Check sheet for the drawn part. Datum: minimum x, y, z corner. Units: mm. A direction names the side the tool comes from. Round coordinates to 2 decimals unless told otherwise and drop trailing zeros. Order: outer loops, then holes, each group sorted by start corner. A loop starts at its lowest first (then second) coordinate and runs counter-clockwise, first axis right, second up. Notation, with made-up numbers: (58.5, 32) -> (102.5, 32) arc R18 cw to (102.5, 40) -> close; hole circle Ø9 at (59.5, 53.5). An arc over 180 degrees is marked (long way). Answer as CSV lines item,"result". Start each with the question number.
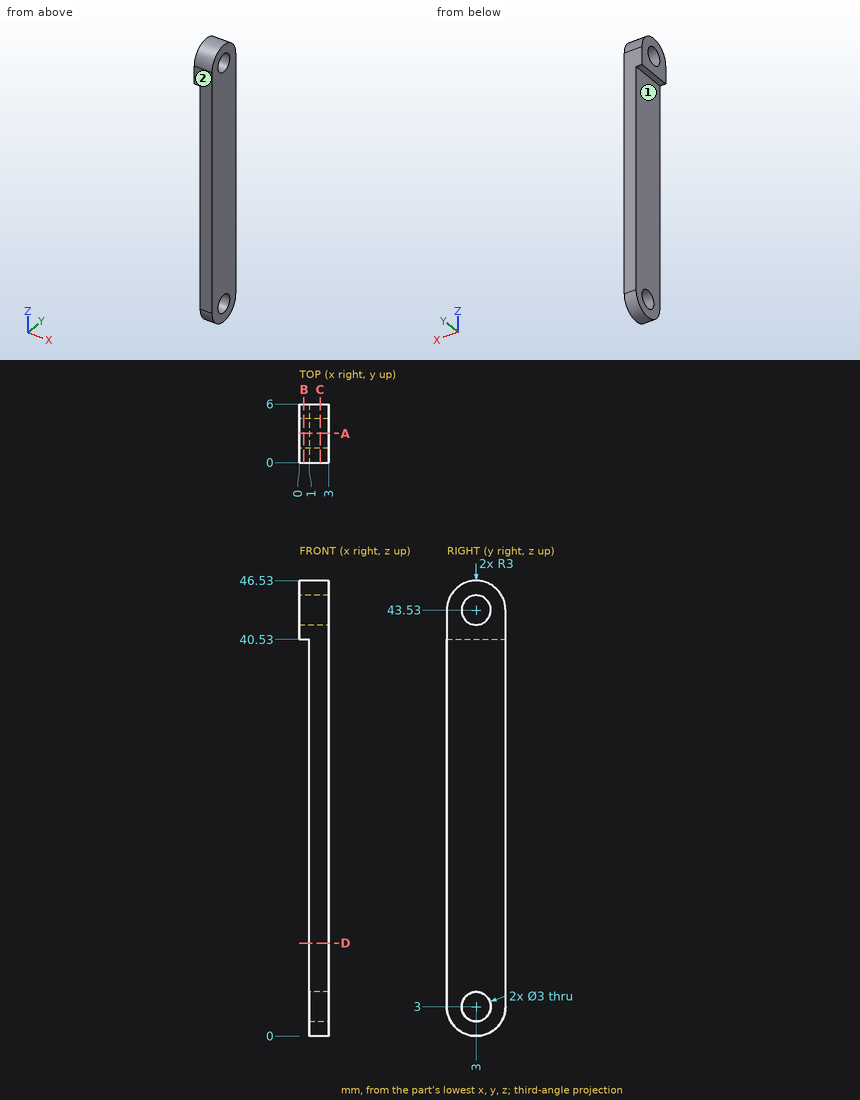
1) Section check A-A on y = 3. Record the cut outline in (x, z), then the cut area to 3 significant figures.
2) Section check B-B on x = 0.45. Record the cut outline in (y, z), then the cut area to 3 significant figures.
3) Depth check by flat-ended pin: pin 1 Ø1 at (x, y) = (1, 1) entering from +Z; pin 2 Ø1.8 at (y, z) = (1.5, 11) entering from -X. Enter the tip coordinate at first touch or a pass-through.
4) Material ranges on line 1 along Z through (x, y) = (1.55, 2.85); line 2 along Z through (x, y) = (1.9, 4.35); line 3 along Z through (x, y) = (0.1, 2.9), recorded low to high.
5) Section check D-D on z = 9.5. Record the cut outline in (x, y).
6) Access from +Z, -Z, +X, -X, +Y, -Y to the whole of each face (thin tool, end or side, straight path). Record for the marked faces 1 and 2.
7) Section check C-C on x = 2.1. Record the cut outline in (y, z).
Solutions:
1,outline,"(0, 40.53) -> (1, 40.53) -> (1, 4.5) -> (3, 4.5) -> (3, 42.03) -> (0, 42.03) -> close; (0, 45.03) -> (3, 45.03) -> (3, 46.53) -> (0, 46.53) -> close; (1, 0) -> (3, 0) -> (3, 1.5) -> (1, 1.5) -> close"
1,area,"84.1 mm^2"
2,outline,"(0, 40.53) -> (6, 40.53) -> (6, 43.53) arc R3 ccw to (0, 43.53) -> close; hole circle Ø3 at (3, 43.53)"
2,area,"25.1 mm^2"
3,pin 1,"stops at z = 46.13"
3,pin 2,"stops at x = 1"
4,line 1,"z = 0 to 1.51, 4.49 to 42.04, 45.02 to 46.53"
4,line 2,"z = 0.32 to 2.35, 3.65 to 42.88, 44.18 to 46.21"
4,line 3,"z = 40.53 to 42.03, 45.03 to 46.53"
5,outline,"(1, 0) -> (3, 0) -> (3, 6) -> (1, 6) -> close"
6,face 1,"-Z, -X, +Y, -Y"
6,face 2,"+Z, -Z, +X, -X, -Y"
7,outline,"(0, 3) arc R3 ccw to (6, 3) -> (6, 43.53) arc R3 ccw to (0, 43.53) -> close; hole circle Ø3 at (3, 3); hole circle Ø3 at (3, 43.53)"
